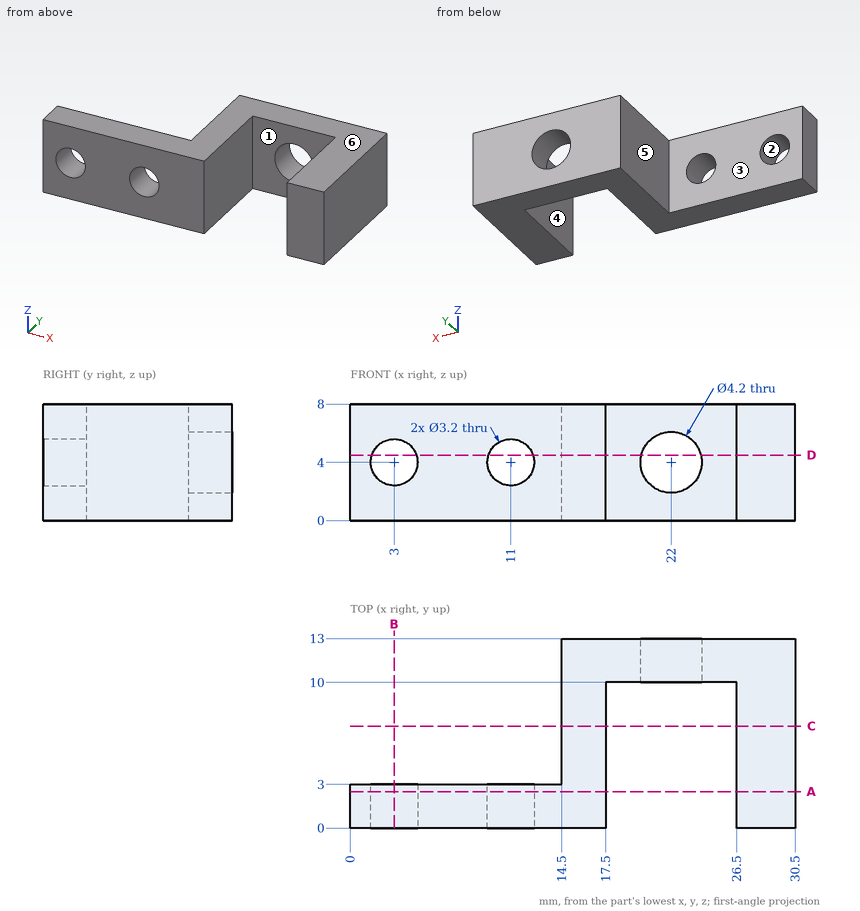
The drawing under review shows one solid part. Ordinate dimensions are in mm from its lowest x, y, z. A direction names the side the tool comes from. Round coordinates to 2 decimals unless told otherwise and drop trailing zeros. Write each loop counter-clockwise with the first axis right and the second up, starting at its lowest first coordinate (ties: lowest second). Pieces come first, ordered by that corner, then holes.
(1) Insertion check: pin 1 (2.5 mm diameter, centred on x = 20, z = 2, fed in from -Y); pin 2 (4 mm diameter, centred on y = 5.5, z = 2.5, fed in from -X). Each pin has a flat end and moves straight along its axis. Give the tip position at first contact, or say it passes through.
(2) We need section D-D on z = 4.5. Give the boundary of the cut face in (x, y), and give its area (3 significant figures).
(3) We need section B-B on x = 3. Give the boundary of the cut face in (y, z), and give its area (3 significant figures).
(4) Wall thickness on L1, parallel to Z at x = 22, y = 11.35; L2, parallel to X at y = 1.3, z = 4; L3, parallel to X at y = 1.75, z = 1.75: over which ranges is each line inside the solid? List them lowest first.
(5) We need section C-C on y = 7. Give the boundary of the cut face in (x, z), and give its area (3 significant figures).
(6) Mouldability with a two-part tool opening along X and no side actions: class the marked faces 4, 5 and 6 as +X half, -X half, draft (parallel to the pull), parting line (faces both ways), or undercut.
(7) We need section A-A on y = 2.5. Give the boundary of the cut face in (x, z), and give its area (3 significant figures).
(8) Machinability: for the marked faces 1, 2 and 3, which of the approach directions +Z, -Z, +X, -X, +Y, -Y give a long, thin tool a straight path to every point of the face, cutting with its end or side? Answer none if there is none.
Findings below:
1. pin 1: stops at y = 10
1. pin 2: stops at x = 14.5
2. outline: (0, 0) - (1.48, 0) - (1.48, 3) - (0, 3) - close; (4.52, 0) - (9.48, 0) - (9.48, 3) - (4.52, 3) - close; (12.52, 0) - (17.5, 0) - (17.5, 10) - (19.96, 10) - (19.96, 13) - (14.5, 13) - (14.5, 3) - (12.52, 3) - close; (24.04, 10) - (26.5, 10) - (26.5, 0) - (30.5, 0) - (30.5, 13) - (24.04, 13) - close
2. area: 131 mm2
3. outline: (0, 0) - (3, 0) - (3, 2.4) - (0, 2.4) - close; (0, 5.6) - (3, 5.6) - (3, 8) - (0, 8) - close
3. area: 14.4 mm2
4. L1: z = 0 to 1.9, 6.1 to 8
4. L2: x = 0 to 1.4, 4.6 to 9.4, 12.6 to 17.5, 26.5 to 30.5
4. L3: x = 0 to 17.5, 26.5 to 30.5
5. outline: (14.5, 0) - (17.5, 0) - (17.5, 8) - (14.5, 8) - close; (26.5, 0) - (30.5, 0) - (30.5, 8) - (26.5, 8) - close
5. area: 56.0 mm2
6. face 4: undercut
6. face 5: -X half
6. face 6: draft
7. outline: (0, 0) - (17.5, 0) - (17.5, 8) - (0, 8) - close; (26.5, 0) - (30.5, 0) - (30.5, 8) - (26.5, 8) - close; hole circle Ø3.2 at (3, 4); hole circle Ø3.2 at (11, 4)
7. area: 156 mm2
8. face 1: +Z, -Z, -Y
8. face 2: +Y, -Y
8. face 3: +Z, -Z, -X, +Y
